```python
from build123d import *

# Parameters (mm, degrees)
F0_W      = 50.8
F0_H      = 76.2
F1_DEPTH  = 50.8
F2_W      = 118.1567646563
F2_H      = 84.5074988902
F3_DEPTH  = 25.4
F7_W      = 50.8
F7_H      = 65.2
F8_DEPTH  = 25.4
F10_DEPTH = 2
F11_R     = 2.5
F12_DEPTH = 25.4
F13_W     = 50.8
F13_H     = 25.4
F14_DEPTH = 25.4
F16_DEPTH = 76.2
F17_W     = 20.6161607057
F17_H     = 59.5903657377
F18_DEPTH = 50.8
F19_W     = 15.1074826717
F19_H     = 54.0688689798
F20_DEPTH = 12.7
F21_DEPTH = 12.7


with BuildPart() as f1:
    # F0 (on Front) → F1 (new body)
    with BuildSketch(Plane.XZ):
        Rectangle(F0_W, F0_H)
    extrude(amount=F1_DEPTH)


with BuildPart() as f3:
    # F2 (on Front) → F3 (new body)
    with BuildSketch(Plane.XZ):
        with Locations((1.1794324964, -5.1696989685)):
            Rectangle(F2_W, F2_H)
    extrude(amount=F3_DEPTH)


with BuildPart() as f3_1:
    # F4: moved
    add(f3.part.moved(Location((0, -6.35, 0))))


with BuildPart() as f1_1:
    add(f1.part)

    # F5: cut F3
    add(f3_1.part, mode=Mode.SUBTRACT)

    # F7 (on face) → F8 (cut)
    with BuildSketch(Plane(origin=(0, 0, 0), x_dir=(-1, 0, 0), z_dir=(0, 1, 0))):
        with Locations((0, -5.5)):
            Rectangle(F7_W, F7_H)
    extrude(amount=-F8_DEPTH, mode=Mode.SUBTRACT)

    # F9 (on face) → F10 (cut)
    with BuildSketch(Plane(origin=(0, -31.75, 0), x_dir=(-1, 0, 0), z_dir=(0, 1, 0))):
        with BuildLine():
            Line((-6, 11.6840504766), (6, 11.6840504766))
            ThreePointArc((6, 11.6840504766), (0, 17.6840504766), (-6, 11.6840504766))
        make_face()
        with BuildLine():
            ThreePointArc((-6, 11.6840504766), (0, 5.6840504766), (6, 11.6840504766))
            Line((6, 11.6840504766), (-6, 11.6840504766))
        make_face()
    extrude(amount=-F10_DEPTH, mode=Mode.SUBTRACT)

    # F11 (on face) → F12 (cut)
    with BuildSketch(Plane(origin=(0, -31.75, 0), x_dir=(-1, 0, 0), z_dir=(0, 1, 0))):
        with Locations((0, 11.6840504766)):
            Circle(F11_R)
    extrude(amount=-F12_DEPTH, mode=Mode.SUBTRACT)

    # F13 (on face) → F14 (cut)
    with BuildSketch(Plane.XZ.offset(50.8)):
        with Locations((0, -25.4)):
            Rectangle(F13_W, F13_H)
    extrude(amount=-F14_DEPTH, mode=Mode.SUBTRACT)

    # F15 (on Front) → F16 (cut)
    with BuildSketch(Plane.XZ):
        Polygon((28.8663152605, 38.4073257446), (8.9931758121, 38.4073257446), (8.9931758121, -14.9972904474), (32.6694212854, -14.9972904474), (32.6694212854, 38.4073257446), align=None)
    extrude(amount=F16_DEPTH, mode=Mode.SUBTRACT)

    # F17 (on Front) → F18 (cut)
    with BuildSketch(Plane.XZ):
        with Locations((-18.4944430366, 13.4912934154)):
            Rectangle(F17_W, F17_H)
    extrude(amount=F18_DEPTH, mode=Mode.SUBTRACT)

    # F19 (on Right) → F20 (cut)
    with BuildSketch(Plane.YZ):
        with Locations((-48.3041740954, 12.0263481513)):
            Rectangle(F19_W, F19_H)
    extrude(amount=-F20_DEPTH, mode=Mode.SUBTRACT)

    # F19 (on Right) → F21 (cut)
    with BuildSketch(Plane.YZ):
        with Locations((-48.3041740954, 12.0263481513)):
            Rectangle(F19_W, F19_H)
    extrude(amount=F21_DEPTH, mode=Mode.SUBTRACT)


solid = f1_1.part
```
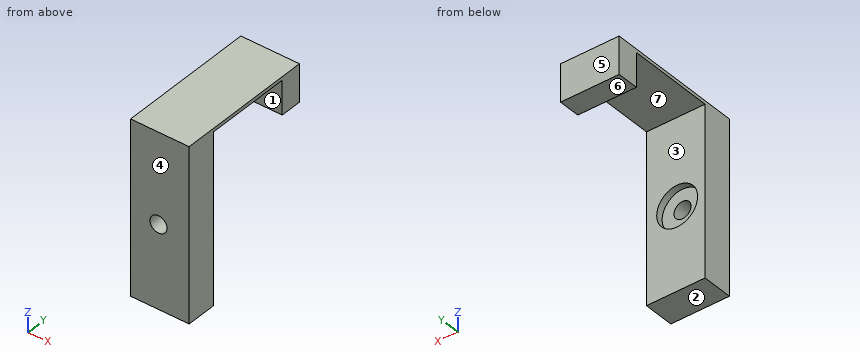
CAD build for the part. Positions are in the model's coordinates, mm. Face numbers are marked on the shaded views. A direction names the side the tool comes from. Round coordinates to 2 decimals unless told otherwise and drop trailing zeros. Order: outer loops, then holes, each group sorted by start corner. A loop starts at its lowest first (then second) coordinate and runs counter-clockwise, first axis right, second up. Notation, with made-up numbers: (51.25, -32.75) - (92.25, -32.75) arc R11 cw to (92.25, -17.75) - close; hole circle Ø6 at (-10, 17). An arc over 180 degrees is marked (long way). Answer in a Markdown table with one row per item. Add a question column.
(1) Probe L1, parallel to Z at x = 0, y = -32.35; L2, parallel to Y at x = 4.5, z = 35; L3, parallel to Z at x = 0, y = -36.75. List the from-to ranges inside material, lowest first. Write a range as [from, to].
(2) Drop flat-ended pins along their axis: pin 1 Ø5 at (x, y) = (4.5, -2.5) entering from -Z; pin 2 Ø1.5 at (x, y) = (5.5, -10.5) entering from -Z; pin 3 Ø6 at (x, z) = (0, 11.68) entering from +Y; pin 4 Ø1.5 at (x, z) = (1, 11.5) entering from +Y. Give the stop position or say it passes through.
(3) Band-saw the part on B-B on x = 0. List the corners of the cut face in (y, z).
(4) Mould opens along Y. For the marked faces 1, 2, 3 and 4 say: +Y half, -Y half, draft (parallel to the pull), parting line (faces both ways), or undercut.
(5) Band-saw the part on C-C on x = 8. List the corners of the cut face in (y, z).
(6) Band-saw the part on A-A on z = 30.5. List the corners of the cut face in (x, y).
(7) 3-axis set-ups, long thin cutter, end or side, ignore diameter. For the marked faces 5, 6 and 7: which of +Z, -Z, +X, -X, +Y, -Y reach the whole face in a straight line?
(8) Band-saw the part on D-D on y = -25.5. List the corners of the cut face in (x, z), and give its area (3 significant figures).
Data:
| question | item | result |
|---|---|---|
| 1 | L1 | z = [-12.7, 5.68], [17.68, 38.1] |
| 1 | L2 | y = [-40.75, -31.75], [-6.35, 0] |
| 1 | L3 | z = [-12.7, 9.18], [14.18, 38.1] |
| 2 | pin 1 | stops at z = 27.1 |
| 2 | pin 2 | stops at z = 37.08 |
| 2 | pin 3 | stops at y = -33.75 |
| 2 | pin 4 | passes through |
| 3 | outline | (-40.75, -12.7) - (-31.75, -12.7) - (-31.75, 5.68) - (-33.75, 5.68) - (-33.75, 9.18) - (-40.75, 9.18) - close; (-40.75, 14.18) - (-33.75, 14.18) - (-33.75, 17.68) - (-31.75, 17.68) - (-31.75, 37.08) - (-6.35, 37.08) - (-6.35, 27.1) - (0, 27.1) - (0, 38.1) - (-40.75, 38.1) - close |
| 4 | face 1 | undercut |
| 4 | face 2 | draft |
| 4 | face 3 | undercut |
| 4 | face 4 | -Y half |
| 5 | outline | (-40.75, -12.7) - (-31.75, -12.7) - (-31.75, 37.08) - (-6.35, 37.08) - (-6.35, 27.1) - (0, 27.1) - (0, 38.1) - (-40.75, 38.1) - close |
| 6 | outline | (-8.19, -40.75) - (8.99, -40.75) - (8.99, -31.75) - (-8.19, -31.75) - close; (-8.19, -6.35) - (8.99, -6.35) - (8.99, 0) - (-8.19, 0) - close |
| 7 | face 5 | +Z, -Z, +X, -X, +Y |
| 7 | face 6 | -Z, +X, -X, +Y |
| 7 | face 7 | -Z, +X, -X |
| 8 | outline | (-8.19, 37.08) - (8.99, 37.08) - (8.99, 38.1) - (-8.19, 38.1) - close |
| 8 | area | 17.5 mm^2 |
